Here's how the part is built. I have some questions about the finished solid (model axes, mm). Round coordinates to 2 decimals unless told otherwise and drop trailing zeros. Write each loop counter-clockwise with the first axis right and the second up, starting at its lowest first coordinate (ties: lowest second). Pieces come first, ordered by that corner, then holes. Notation, with made-up numbers: (52, -31) - (104, -31) arc R24 ccw to (104, -7) - close; hole circle Ø7 at (-36.75, 5.5). An arc over 180 degrees is marked (long way). Use one line per item in the form item = value. Start each with the question number.
1. I want a section at B-B, the plane z = 12. List the corners of the cut face in (x, y) for me (3 decimals), plus the area to 3 significant figures.
2. Will these pins go through, and if not, where does the flat tip stop? pin 1 (4 mm diameter, centred on x = -43.5, z = 7, fed in from +Y); pin 2 (3 mm diameter, centred on x = -37.5, y = 239.5, fed in from -Z).
3. If I drill on line 1 along X through (y, z) = (494.5, 2.25); line 2 along Y through (x, z) = (-36.5, 2.5); line 3 along Y through (x, z) = (-36, 2.75), over which ranges is the centre line in solid material (lowest first)?
4. I want a section at A-A, the plane y = 431. List the corners of the cut face in (x, z) for me.
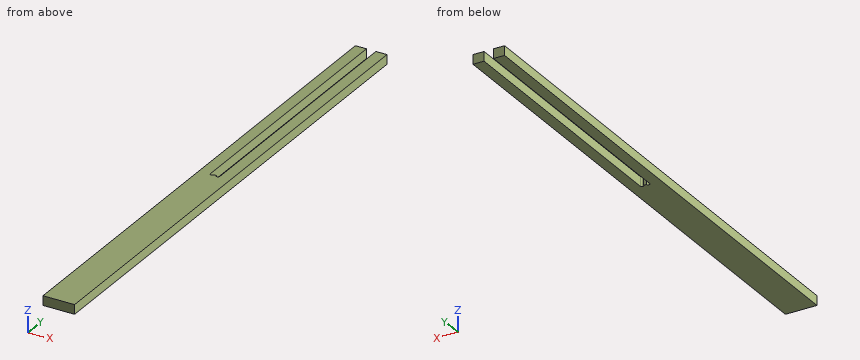
```python
from build123d import *

# Parameters (mm, degrees)
ESTRUSIONE_ESTRUSIONE1_DEPTH = 18


with BuildPart() as part:
    # Schizzo1 → Estrusione-Estrusione1 (new body)
    with BuildSketch(Plane.XY):
        with BuildLine():
            Line((-51.222222222, 825), (-51.222222222, 325))
            ThreePointArc((-51.222222222, 325), (-48.047222222, 321.825), (-44.872222222, 325))
            Line((-44.872222222, 325), (-39.572222222, 325))
            ThreePointArc((-39.572222222, 325), (-36.397222222, 321.825), (-33.222222222, 325))
            Line((-33.222222222, 325), (-33.222222222, 825))
            Line((-33.222222222, 825), (-12.222222222, 825))
            Line((-12.222222222, 825), (-12.222222222, -175))
            Line((-12.222222222, -175), (-72.222222222, -175))
            Line((-72.222222222, -175), (-72.222222222, 825))
            Line((-72.222222222, 825), (-51.222222222, 825))
        make_face()
    extrude(amount=ESTRUSIONE_ESTRUSIONE1_DEPTH)


solid = part.part
```
Model answer:
q1.outline = (-72.222, -175) - (-12.222, -175) - (-12.222, 825) - (-33.222, 825) - (-33.222, 325) arc R3.175 cw to (-39.572, 325) - (-44.872, 325) arc R3.175 cw to (-51.222, 325) - (-51.222, 825) - (-72.222, 825) - close
q1.area = 51,000 mm2
q2.pin_1 = 325
q2.pin_2 = 0
q3.line_1 = -72.22 to -51.22, -33.22 to -12.22
q3.line_2 = -175 to 321.83
q3.line_3 = -175 to 321.85
q4.outline = (-72.22, 0) - (-51.22, 0) - (-51.22, 18) - (-72.22, 18) - close; (-33.22, 0) - (-12.22, 0) - (-12.22, 18) - (-33.22, 18) - close
